from build123d import *

# Parameters (mm, degrees)
ESQUISSE1_R             = 75
ESQUISSE1_R_2           = 52.5
BOSS_EXTRU_1_DEPTH      = 30
ESQUISSE2_R             = 52.5
ESQUISSE2_R_2           = 37.5
BOSS_EXTRU_2_DEPTH      = 19.5
ESQUISSE3_R             = 42.5
ESQUISSE3_R_2           = 37.5
BOSS_EXTRU_3_DEPTH      = 5
ESQUISSE4_R             = 75
ESQUISSE4_R_2           = 37.5
ENL_V_MAT_EXTRU_1_DEPTH = 17


with BuildPart() as part:
    # Esquisse1 → Boss.-Extru.1 (new body)
    with BuildSketch(Plane.XY):
        Circle(ESQUISSE1_R)
        Circle(ESQUISSE1_R_2, mode=Mode.SUBTRACT)
    extrude(amount=BOSS_EXTRU_1_DEPTH)

    # Esquisse2 → Boss.-Extru.2 (add)
    with BuildSketch(Plane.XY.offset(30)):
        Circle(ESQUISSE2_R)
        Circle(ESQUISSE2_R_2, mode=Mode.SUBTRACT)
    extrude(amount=-BOSS_EXTRU_2_DEPTH)

    # Esquisse3 → Boss.-Extru.3 (add)
    with BuildSketch(Plane(origin=(0, 0, 10.5), x_dir=(-1, 0, 0), z_dir=(0, 0, -1))):
        with Locations(Location((0, 0, 0), (0, 0, 180))):
            Circle(ESQUISSE3_R)
        with Locations(Location((0, 0, 0), (0, 0, 180))):
            Circle(ESQUISSE3_R_2, mode=Mode.SUBTRACT)
    extrude(amount=BOSS_EXTRU_3_DEPTH)

    # Esquisse4 → Enlèv. mat.-Extru.1 (cut)
    with BuildSketch(Plane.XY.offset(30)):
        Circle(ESQUISSE4_R)
        Circle(ESQUISSE4_R_2, mode=Mode.SUBTRACT)
    extrude(amount=-ENL_V_MAT_EXTRU_1_DEPTH, mode=Mode.SUBTRACT)


solid = part.part
Read the model definition and answer for the solid it produces. Units are mm, in the model's axes. A direction names the side the tool comes from. Coordinates: 2 decimals unless noted, no trailing zeros. Loops run counter-clockwise (first coordinate to the right, second up) from the corner with the lowest first, then second, coordinate; pieces in that order, holes last. Notation, with made-up numbers: (40.5, -16.5) - (98.5, -16.5) arc R21 ccw to (98.5, 14.5) - close; hole circle Ø8 at (-20.5, -22). An arc over 180 degrees is marked (long way). Answer in a Markdown table with one row per item.
Q1. Find section D-D on x = -46. Write down the section's boundary in (y, z).
Here are the results:
| item | result |
|---|---|
| outline | (-59.24, 0) - (-25.3, 0) - (-25.3, 10.5) - (25.3, 10.5) - (25.3, 0) - (59.24, 0) - (59.24, 13) - (-59.24, 13) - close |
Q2. For faces 4 (the flat face through (15.6, 34.4, 13)), 5 (the cylindrical face through (50.076, 15.77, 5.176)), determine the directions among +Z, -Z, +X, -X, +Y, -Y from which every point of the face is accessible in a straight line to the end or side of a thin tool.
Here are the results:
| item | result |
|---|---|
| face 4 | +Z, +X, -X, +Y, -Y |
| face 5 | -Z |
Q3. Straight lines are drawn through the part: line 1 along Y through (x, z) = (0, 5.75); line 2 along X through (y, z) = (-25, 7.75); line 3 along Y through (x, z) = (-20, 8). For each, find the intervals that lie inside material, in ascending order. Write a range as [from, to].
Here are the results:
| item | result |
|---|---|
| line 1 | y = [-75, -52.5], [-42.5, -37.5], [37.5, 42.5], [52.5, 75] |
| line 2 | x = [-70.71, -46.17], [-34.37, -27.95], [27.95, 34.37], [46.17, 70.71] |
| line 3 | y = [-72.28, -48.54], [-37.5, -31.72], [31.72, 37.5], [48.54, 72.28] |
Q4. The mould has two halves that part along Y. Classify faces 1 (the flat face through (16, 51, 0)), 2 (the cylindrical face through (-9.764, 74.362, 6.409)), 3 (the flat face through (0, 38, 5.5)): pulls with the +Y half, pulls with the -Y half, needs draft (parallel to the pull), parting line crosses it, or undercut.
Here are the results:
| item | result |
|---|---|
| face 1 | needs draft |
| face 2 | parting line crosses it |
| face 3 | undercut |
Q5. Given P1, Ø6, axis at x = -12, y = 29.5, coming from the +Z side; P2, Ø5, axis at y = 24.5, z = 10, coming from the -X side; P3, Ø3, axis at y = -41.5, z = 3, coming from the -X side; P4, Ø4, axis at x = 50, z = 3, coming from the -Y side, each flat-ended and moving along its own axis, determine where each tip first touches the part or whether it passes through.
Here are the results:
| item | result |
|---|---|
| P1 | passes through |
| P2 | stops at x = -71.7 |
| P3 | stops at x = -63.44 |
| P4 | stops at y = -57.63 |
Q6. Find section B-B on y = 0. Write down the section's boundary in (x, z).
Here are the results:
| item | result |
|---|---|
| outline | (-75, 0) - (-52.5, 0) - (-52.5, 10.5) - (-42.5, 10.5) - (-42.5, 5.5) - (-37.5, 5.5) - (-37.5, 13) - (-75, 13) - close; (37.5, 5.5) - (42.5, 5.5) - (42.5, 10.5) - (52.5, 10.5) - (52.5, 0) - (75, 0) - (75, 13) - (37.5, 13) - close |
Q7. Find section A-A on z = 7.5. Write down the section's boundary in (x, y).
Here are the results:
| item | result |
|---|---|
| outline | circle Ø150 at (0, 0); circle Ø85 at (0, 0); hole circle Ø105 at (0, 0); hole circle Ø75 at (0, 0) |
